Here's the drawing with two shaded views (mm, measured from the low corner). I have some questions. A direction names the side the tool comes from. Coordinates: 2 decimals unless noted, no trailing zeros. Write each loop counter-clockwise with the first axis right and the second up, starting at its lowest first coordinate (ties: lowest second). Pieces come first, ordered by that corner, then holes. Notation, with made-up numbers: (-17.75, 67.25) -> (36.25, 67.25) arc R25 cw to (36.25, 80.25) -> close; hole circle Ø8 at (45.25, 30.5). An arc over 180 degrees is marked (long way). Put each result on its own line as item: value. Start each with the question number.
Item 1: If we mould it in two halves opening along Y, with no side actions, what happens to the marked faces 4, 5 and 6? For each: released by +Y, released by -Y, zero draft, split by the parting line, or undercut.
Item 2: I want a section at C-C, the plane x = 3.75. List the corners of the cut face in (y, z) for me, then the cut area to 3 significant figures.
Item 3: For pin 1 (3 mm diameter, centred on x = 4.5, z = 15, fed in from +Y); pin 2 (7.5 mm diameter, centred on x = 7.5, y = 10, fed in from -Z); pin 3 (1.2 mm diameter, centred on y = 8.5, z = 4, fed in from -X); pin 4 (1.2 mm diameter, centred on y = 7.5, z = 5, fed in from +X), each with a flat end and sliding along its axis, tell me the tip position at first contact or that it passes through.
Item 4: On a 3-axis mill with a long thin cutter (end or side, diameter ignored), from which of +Z, -Z, +X, -X, +Y, -Y can I reach the whole of each face in a straight line? I mean the marked faces 1, 2 and 3. Say none if no direction works.
Item 5: I want a section at D-D, the plane y = 7.75. List the corners of the cut face in (x, z) for me (1 decimal).
Item 6: I need wall thicknesses on line 1 (Y direction, x = 8.35, z = 18.5); line 2 (Y direction, x = 8.35, z = 1.3) (1 decimal); line 3 (Z direction, x = 5, y = 7.25). Which ranges of each line are inside material? Lowest first, please. Write a range as [from, to].
Item 7: I want a section at A-A, the plane y = 11.75. List the corners of the cut face in (x, z) for me, then the cut area to 3 significant figures.
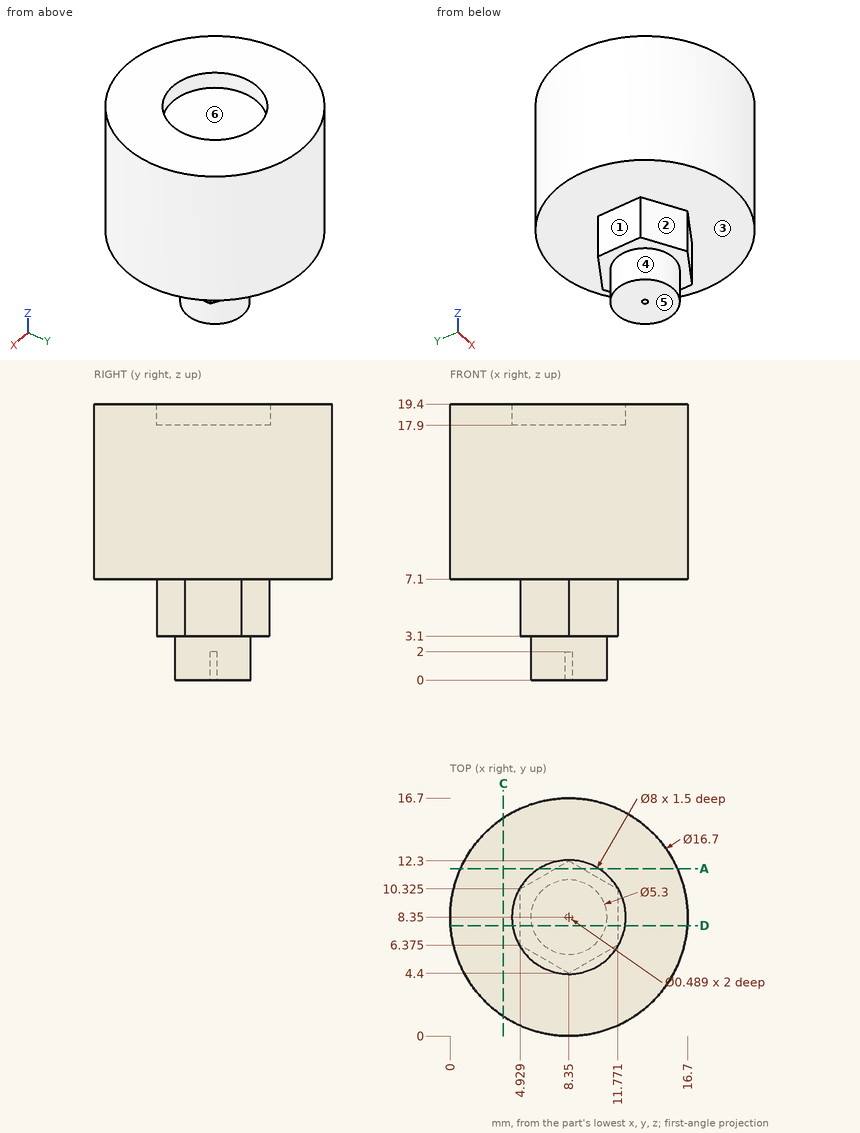
Calculated:
1. face 4: split by the parting line
1. face 5: zero draft
1. face 6: undercut
2. outline: (1.38, 7.1) -> (15.32, 7.1) -> (15.32, 19.4) -> (1.38, 19.4) -> close
2. area: 171 mm2
3. pin 1: stops at y = 16.36
3. pin 2: stops at z = 0
3. pin 3: stops at x = 4.93
3. pin 4: stops at x = 11.77
4. face 1: -Z, -X, +Y, -Y
4. face 2: -Z, -X, -Y
4. face 3: -Z
5. outline: (0, 7.1) -> (4.9, 7.1) -> (4.9, 3.1) -> (5.8, 3.1) -> (5.8, 0) -> (10.9, 0) -> (10.9, 3.1) -> (11.8, 3.1) -> (11.8, 7.1) -> (16.7, 7.1) -> (16.7, 19.4) -> (12.3, 19.4) -> (12.3, 17.9) -> (4.4, 17.9) -> (4.4, 19.4) -> (0, 19.4) -> close
6. line 1: y = [0, 4.35], [12.35, 16.7]
6. line 2: y = [5.7, 8.1], [8.6, 11]
6. line 3: z = [3.1, 17.9]
7. outline: (0.72, 7.1) -> (7.4, 7.1) -> (7.4, 3.1) -> (9.3, 3.1) -> (9.3, 7.1) -> (15.98, 7.1) -> (15.98, 19.4) -> (10.46, 19.4) -> (10.46, 17.9) -> (6.24, 17.9) -> (6.24, 19.4) -> (0.72, 19.4) -> close
7. area: 189 mm2
